from build123d import *

# Parameters (mm, degrees)
F1_DEPTH = 38.1
F3_DEPTH = 19.05
F5_DEPTH = 19.05


with BuildPart() as f1:
    # F0 (on Front) → F1 (new body)
    with BuildSketch(Plane.XZ):
        Polygon((457.2, 0), (0, 0), (3.333318, -38.1), (453.866682, -38.1), align=None)
    extrude(amount=F1_DEPTH)

    # F2 (on face) → F3 (cut)
    with BuildSketch(Plane.XZ.offset(38.1)):
        Polygon((457.2, 0), (418.954464, 0), (415.621146, -38.1), (453.866682, -38.1), align=None)
    extrude(amount=-F3_DEPTH, mode=Mode.SUBTRACT)

    # F4 (on face) → F5 (cut)
    with BuildSketch(Plane.XZ.offset(38.1)):
        Polygon((41.578854, -38.1), (38.245536, 0), (0, 0), (3.333318, -38.1), align=None)
    extrude(amount=-F5_DEPTH, mode=Mode.SUBTRACT)


solid = f1.part
Model file for the job. Use its own axes, mm. A direction names the side the tool comes from. Give positions to 0.01 mm unless a question says otherwise; leave off trailing zeros. Write each loop counter-clockwise with the first axis right and the second up, starting at its lowest first coordinate (ties: lowest second). Pieces come first, ordered by that corner, then holes. Notation, with made-up numbers: M 31,48 L 65,48 A26 ccw 65,69 Z; hole C -4.75,88 d4. An arc over 180 degrees is marked long. One line per item, written item: value. Start each with the question number.
Q1. Saw through at A-A, the plane z = -19. Write the cut outline in (x, y), plus the area to 3 significant figures.
Q2. Saw through at C-C, the plane x = 33.5. Write the cut outline in (y, z).
Q3. Drop flat-ended pins along their axis: pin 1 Ø1 at (y, z) = (-15.5, -33) entering from -X; pin 2 Ø2 at (x, z) = (294.5, -6) entering from +Y; pin 3 Ø5 at (y, z) = (-9.5, -23) entering from +X; pin 4 Ø2 at (y, z) = (-32, -24.5) entering from +X. Give the stop position or say it passes through.
Q4. 3-axis set-ups, long thin cutter, end or side, ignore diameter. For faces 1 (the flat face through (417.31, -28.71, -18.78)), 2 (the flat face through (1.643, -9.392, -18.783)), 3 (the flat face through (39.936, -28.708, -19.317)): which of +Z, -Z, +X, -X, +Y, -Y reach the whole face in a straight line?
Q5. Probe probe 1 along Y at (x, z) = (424, -36.5); probe 2 along X at (y, z) = (-34.5, -32); probe 3 along X at (y, z) = (-11, -20). List the from-to ranges inside material, lowest first. Write a range as [from, to].
Q6. Saw through at B-B, the plane y = -26. Write the cut outline in (x, z), plus the area to 3 significant figures.
Output values:
1. outline: M 1.66,-19.05 L 39.91,-19.05 L 39.91,-38.1 L 417.29,-38.1 L 417.29,-19.05 L 455.54,-19.05 L 455.54,0 L 1.66,0 Z
1. area: 15,800 mm²
2. outline: M -19.05,-38.1 L 0,-38.1 L 0,0 L -19.05,0 Z
3. pin 1: stops at x = 2.84
3. pin 2: stops at y = 0
3. pin 3: stops at x = 455.41
3. pin 4: stops at x = 416.9
4. face 1: -Z, +X, -Y
4. face 2: -Z, -X, +Y, -Y
4. face 3: -Z, -X, -Y
5. probe 1: y = [-19.05, 0]
5. probe 2: x = [41.05, 416.15]
5. probe 3: x = [1.75, 455.45]
6. outline: M 38.25,0 L 41.58,-38.1 L 415.62,-38.1 L 418.95,0 Z
6. area: 14,400 mm²
